Here's how the part is built. I have some questions about the finished solid (model axes, mm). A direction names the side the tool comes from. Round coordinates to 2 decimals unless told otherwise and drop trailing zeros. Loops run counter-clockwise (first coordinate to the right, second up) from the corner with the lowest first, then second, coordinate; pieces in that order, holes last. Notation, with made-up numbers: M -30.75,69.25 L 16.25,69.25 A32 cw 16.25,102.25 Z; hole C -32,18 d8. An arc over 180 degrees is marked long. Write each question's results on one line, items separated by ' | '. Start each with the question number.
```python
from build123d import *

# Parameters (mm, degrees)
SKETCH_2_W                = 40
SKETCH_2_H                = 39
EXTRUDE_1_DEPTH           = 10
FILLET_1_R                = 1
SKETCH_6_R                = 4
CUT_EXTRUDE_1_DEPTH       = 2
HOLE_WIZARD_2_0_2_2_D     = 2
HOLE_WIZARD_2_0_2_2_DEPTH = 10
HOLE_WIZARD_2_0_2_2_TIP   = 0.600860619
EXTRUDE_START             = -8
SKETCH_16_W               = 7
SKETCH_16_H               = 19
SKETCH_16_R               = 2
EXTRUDE_2_DEPTH           = 3
SKETCH_17_R               = 6.5
EXTRUDE_3_DEPTH           = 1.5
SKETCH_18_R               = 5
EXTRUDE_4_DEPTH           = 0.5
SKETCH_19_R               = 3
EXTRUDE_5_DEPTH           = 4
FILLET_2_R                = 1
HOLE_WIZARD_M3_1_D        = 2.5
HOLE_WIZARD_M3_1_DEPTH    = 5.55
HOLE_WIZARD_M3_1_TIP      = 0.751075774
SKETCH_22_W               = 7.5
SKETCH_22_H               = 5
EXTRUDE_6_DEPTH           = 1
LOFT_1_OUTLINE_W          = 3.5
LOFT_1_OUTLINE_H          = 6
LOFT_1_DEPTH              = 4.5
LOFT_1_DRAFT              = -3.1798301
SKETCH_26_R               = 0.9
EXTRUDE_8_DEPTH           = 5


# Read off the part's stored shape, not the designer's step: 放样1
with BuildPart() as part:
    # 草图2 → 凸台-拉伸1 (new, symmetric)
    with BuildSketch(Plane.XY):
        with Locations((20, -19.5)):
            Rectangle(SKETCH_2_W, SKETCH_2_H)
    extrude(amount=EXTRUDE_1_DEPTH, both=True)

    # 圆角1
    fillet_1_edges = [part.edges().sort_by_distance(p)[0] for p in [
        (40, -19.5, 10),
        (20, 0, 10),
        (0, -19.5, 10),
        (20, 0, -10),
        (40, -19.5, -10),
        (20, -39, -10),
        (0, -19.5, -10),
        (20, -39, 10),
        (0, 0, 0),
        (40, 0, 0),
        (40, -39, 0),
        (0, -39, 0),
    ]]
    fillet(fillet_1_edges, radius=FILLET_1_R)

    # 草图6 → 切除-拉伸1 (cut)
    with BuildSketch(Plane.XZ):
        with Locations((0, 10)):
            Circle(SKETCH_6_R)
        with Locations((40, 10)):
            Circle(SKETCH_6_R)
        with Locations((40, -10)):
            Circle(SKETCH_6_R)
        with Locations((0, -10)):
            Circle(SKETCH_6_R)
    extrude(amount=CUT_EXTRUDE_1_DEPTH, mode=Mode.SUBTRACT)

    # Ø2.0 (2) 直径孔2
    with Locations(Plane(origin=(0, -39, 0), x_dir=(-1, 0, 0), z_dir=(0, -1, 0))):
        with Locations((-37.5, 7.5), (-37.5, -7.5), (-2.5, 7.5), (-2.5, -7.5)):
            Hole(HOLE_WIZARD_2_0_2_2_D / 2, depth=HOLE_WIZARD_2_0_2_2_DEPTH)
            with Locations((0, 0, -(HOLE_WIZARD_2_0_2_2_DEPTH + HOLE_WIZARD_2_0_2_2_TIP / 2))):  # 118° drill point
                Cone(0, HOLE_WIZARD_2_0_2_2_D / 2, HOLE_WIZARD_2_0_2_2_TIP, mode=Mode.SUBTRACT)

    # 草图16 → 凸台-拉伸2 (add)
    # profile 1 of 2: a face of its own
    with BuildSketch(Plane(origin=(0, 0, 0), x_dir=(1, 0, 0), z_dir=(0, 1, 0)).offset(EXTRUDE_START)):
        with Locations((-3.5, 0)):
            Rectangle(SKETCH_16_W, SKETCH_16_H)
        with Locations(Location((-4, -5, 0), (0, 0, 270))):
            Circle(SKETCH_16_R, mode=Mode.SUBTRACT)
        with Locations(Location((-4, 5, 0), (0, 0, 270))):
            Circle(SKETCH_16_R, mode=Mode.SUBTRACT)
    # profile 2 of 2: a face of its own
    with BuildSketch(Plane(origin=(0, 0, 0), x_dir=(1, 0, 0), z_dir=(0, 1, 0)).offset(EXTRUDE_START)):
        with Locations((43.5, 0)):
            Rectangle(SKETCH_16_W, SKETCH_16_H)
        with Locations(Location((44, 5, 0), (0, 0, 90))):
            Circle(SKETCH_16_R, mode=Mode.SUBTRACT)
        with Locations(Location((44, -5, 0), (0, 0, 90))):
            Circle(SKETCH_16_R, mode=Mode.SUBTRACT)
    extrude(amount=-EXTRUDE_2_DEPTH)

    # 草图17 → 凸台-拉伸3 (add)
    with BuildSketch(Plane(origin=(0, 0, 0), x_dir=(1, 0, 0), z_dir=(0, 1, 0))):
        with Locations(Location((10, 0, 0), (0, 0, 90))):
            Circle(SKETCH_17_R)
    extrude(amount=EXTRUDE_3_DEPTH)

    # 草图18 → 凸台-拉伸4 (add)
    with BuildSketch(Plane(origin=(0, 1.5, 0), x_dir=(1, 0, 0), z_dir=(0, 1, 0))):
        with Locations(Location((10, 0, 0), (0, 0, 270))):
            Circle(SKETCH_18_R)
    extrude(amount=EXTRUDE_4_DEPTH)

    # 草图19 → 凸台-拉伸5 (add)
    with BuildSketch(Plane(origin=(0, 2, 0), x_dir=(1, 0, 0), z_dir=(0, 1, 0))):
        with Locations(Location((10, 0, 0), (0, 0, 270))):
            Circle(SKETCH_19_R)
    extrude(amount=EXTRUDE_5_DEPTH)

    # 圆角2
    fillet_2_edges = [part.edges().sort_by_distance(p)[0] for p in [
        (-7, -9.5, 9.5),
        (-7, -9.5, -9.5),
        (47, -9.5, 9.5),
        (47, -9.5, -9.5),
    ]]
    fillet(fillet_2_edges, radius=FILLET_2_R)

    # M3 螺纹孔1
    with Locations(Plane(origin=(0, 6, 0), x_dir=(1, 0, 0), z_dir=(0, 1, 0))):
        with Locations((10, 0)):
            Hole(HOLE_WIZARD_M3_1_D / 2, depth=HOLE_WIZARD_M3_1_DEPTH)
            with Locations((0, 0, -(HOLE_WIZARD_M3_1_DEPTH + HOLE_WIZARD_M3_1_TIP / 2))):  # 118° drill point
                Cone(0, HOLE_WIZARD_M3_1_D / 2, HOLE_WIZARD_M3_1_TIP, mode=Mode.SUBTRACT)

    # 草图22 → 凸台-拉伸6 (add)
    with BuildSketch(Plane.ZY):
        with Locations((0, -34.5)):
            Rectangle(SKETCH_22_W, SKETCH_22_H)
    extrude(amount=EXTRUDE_6_DEPTH)


with BuildPart() as loft_1_tool:
    # 放样1 outline → 放样1 (with draft: the straight prism first)
    with BuildSketch(Plane.YZ.offset(-5.5)):
        with Locations((-34.5, 0)):
            Rectangle(LOFT_1_OUTLINE_W, LOFT_1_OUTLINE_H)
    extrude(amount=LOFT_1_DEPTH)
    # 放样1: the draft: its side faces are tilted about the plane it starts from
    loft_1_sides = [loft_1_tool.faces().sort_by_distance(p)[0] for p in [
        (-3.25, -36.25, 0),
        (-3.25, -34.5, -3),
        (-3.25, -32.75, 0),
        (-3.25, -34.5, 3),
    ]]
    draft(loft_1_sides, Plane.YZ.offset(-5.5), LOFT_1_DRAFT)


with BuildPart() as part_1:
    add(part.part)

    # 放样1: add loft_1_tool
    add(loft_1_tool.part)

    # 草图26 → 凸台-拉伸8 (add)
    with BuildSketch(Plane.ZY.offset(5.5)):
        with Locations((-2, -34.5)):
            Circle(SKETCH_26_R)
        with Locations((0, -34.5)):
            Circle(SKETCH_26_R)
        with Locations((2, -34.5)):
            Circle(SKETCH_26_R)
    extrude(amount=EXTRUDE_8_DEPTH)


solid = part_1.part
```
Item 1: I'm going to push flat-ended pins straight in: pin 1 (5.5 mm diameter, centred on x = 43, z = 1.5, fed in from -Y); pin 2 (4 mm diameter, centred on y = 1, z = 5, fed in from +X); pin 3 (8 mm diameter, centred on y = -11, z = -0.5, fed in from -X). Where does each tip first touch, or does it pass through?
Item 2: I need wall thicknesses on L1, parallel to X at y = -8.95, z = -5; L2, parallel to Z at x = 2.5, y = -33.5; L3, parallel to X at y = -32.25, z = -7.5. Which ranges of each line are inside material? Lowest first, please.
Item 3: Which directions (+Z, -Z, +X, -X, +Y, -Y) give clear straight access to the entire face, cutting with the end or side of a thin tool? Please do faces 5 (the face through (38, -2, 8)), 6 (the face through (37.203, -0.986, -7.141)), 7 (the face through (2, -2, -8)).
Item 4: If we section it at A-A on y = -30.5: Please give me the cut outline in (x, z).
Item 5: If we section it at C-C on x = -3: Please give me the cut outline in (y, z).
Item 6: If we section it at B-B on y = -15: Please give me the cut outline in (x, z).
Item 7: If we mould it in two halves opening along Z, with no side actions, what happens to faces 1 (the face through (43, -9, -9.5)), 2 (the face through (2.34, -28.503, 7.567)), 3 (the face through (-1, -32.2, -0.1)), 4 (the face through (-7.96, -33.74, 2.48))? For each: released by +Z, released by -Z, zero draft, split by the parting line, or undercut.
Numbers:
1) pin 1: y = -11 | pin 2: x = 40 | pin 3: x = -7
2) L1: -7 to -6, -2 to 42, 46 to 47 | L2: -10 to -8.5, -6.5 to 6.5, 8.5 to 10 | L3: 0 to 1.5, 3.5 to 36.5, 38.5 to 40
3) face 5: +Z, +X, +Y | face 6: -Z, +X, +Y | face 7: -Z, -X, +Y
4) outline: M 0,-9 A1 ccw 1,-10 L 39,-10 A1 ccw 40,-9 L 40,9 A1 ccw 39,10 L 1,10 A1 ccw 0,9 Z; hole C 2.5,-7.5 d2; hole C 2.5,7.5 d2; hole C 37.5,-7.5 d2; hole C 37.5,7.5 d2
5) outline: M -36.39,-3.14 L -32.61,-3.14 L -32.61,3.14 L -36.39,3.14 Z; M -11,-9.5 L -8,-9.5 L -8,-6.73 L -11,-6.73 Z; M -11,-3.27 L -8,-3.27 L -8,3.27 L -11,3.27 Z; M -11,6.73 L -8,6.73 L -8,9.5 L -11,9.5 Z
6) outline: M 0,-9 A1 ccw 1,-10 L 39,-10 A1 ccw 40,-9 L 40,9 A1 ccw 39,10 L 1,10 A1 ccw 0,9 Z
7) face 1: released by -Z | face 2: undercut | face 3: zero draft | face 4: undercut
